For this review, take the finished solid that the model builds, in its own axes (mm). Face numbers are marked on the shaded views. A direction names the side the tool comes from. Coordinates: 2 decimals unless noted, no trailing zeros. Order: outer loops, then holes, each group sorted by start corner. A loop starts at its lowest first (then second) coordinate and runs counter-clockwise, first axis right, second up. Notation, with made-up numbers: M 29.25,11 L 82.25,11 A31 ccw 82.25,36 Z; hole C 26,48 d9. An arc over 180 degrees is marked long. Use CSV: the item, a comma, the result in double quotes.
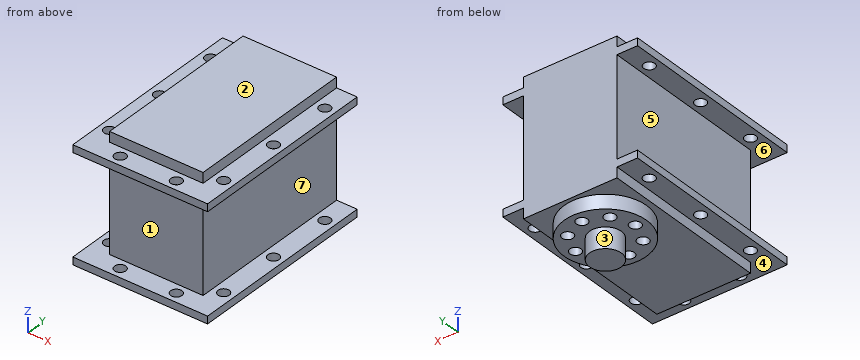
```python
from build123d import *

# Parameters (mm, degrees)
SKETCH1_W           = 25
SKETCH1_H           = 45.5
BOSS_EXTRUDE1_DEPTH = 36
BOSS_EXTRUDE2_START = -2.75
SKETCH2_W           = 36
SKETCH2_H           = 51
SKETCH2_R           = 1.5
BOSS_EXTRUDE2_DEPTH = 2
SKETCH3_R           = 11
BOSS_EXTRUDE3_DEPTH = 3.75
SKETCH4_R           = 1.5
CUT_EXTRUDE1_DEPTH  = 3.75
SKETCH5_R           = 4.25
BOSS_EXTRUDE4_DEPTH = 5.5
BOSS_EXTRUDE5_START = -4.75
SKETCH6_W           = 36
SKETCH6_H           = 51
SKETCH6_R           = 1.5
BOSS_EXTRUDE5_DEPTH = 2


with BuildPart() as part:
    # Sketch1 → Boss-Extrude1 (new body)
    with BuildSketch(Plane.XY):
        Rectangle(SKETCH1_W, SKETCH1_H)
    extrude(amount=BOSS_EXTRUDE1_DEPTH)

    # Sketch2 → Boss-Extrude2 (add)
    with BuildSketch(Plane(origin=(0, 0, 0), x_dir=(-1, 0, 0), z_dir=(0, 0, -1)).offset(BOSS_EXTRUDE2_START)):
        with Locations((0, -2.75)):
            Rectangle(SKETCH2_W, SKETCH2_H)
        with Locations((-15.25, 15.25)):
            Circle(SKETCH2_R, mode=Mode.SUBTRACT)
        with Locations((-15.25, -2.25)):
            Circle(SKETCH2_R, mode=Mode.SUBTRACT)
        with Locations((-15.25, -19.25)):
            Circle(SKETCH2_R, mode=Mode.SUBTRACT)
        with Locations((-7.5, -25.5)):
            Circle(SKETCH2_R, mode=Mode.SUBTRACT)
        with Locations((7.5, -25.5)):
            Circle(SKETCH2_R, mode=Mode.SUBTRACT)
        with Locations((15.25, -19.25)):
            Circle(SKETCH2_R, mode=Mode.SUBTRACT)
        with Locations((15.25, -2.25)):
            Circle(SKETCH2_R, mode=Mode.SUBTRACT)
        with Locations((15.25, 15.25)):
            Circle(SKETCH2_R, mode=Mode.SUBTRACT)
    extrude(amount=-BOSS_EXTRUDE2_DEPTH)

    # Sketch3 → Boss-Extrude3 (add)
    with BuildSketch(Plane(origin=(0, 0, 0), x_dir=(-1, 0, 0), z_dir=(0, 0, -1))):
        with Locations((0, 10.75)):
            Circle(SKETCH3_R)
    extrude(amount=BOSS_EXTRUDE3_DEPTH)

    # Sketch4 → Cut-Extrude1 (cut)
    with BuildSketch(Plane(origin=(0, 0, -3.75), x_dir=(-1, 0, 0), z_dir=(0, 0, -1))):
        with Locations((0, 18.75)):
            Circle(SKETCH4_R)
        with Locations((-5.656854249, 16.406854249)):
            Circle(SKETCH4_R)
        with Locations((-8, 10.75)):
            Circle(SKETCH4_R)
        with Locations((-5.656854249, 5.093145751)):
            Circle(SKETCH4_R)
        with Locations((0, 2.75)):
            Circle(SKETCH4_R)
        with Locations((5.656854249, 5.093145751)):
            Circle(SKETCH4_R)
        with Locations((8, 10.75)):
            Circle(SKETCH4_R)
        with Locations((5.656854249, 16.406854249)):
            Circle(SKETCH4_R)
    extrude(amount=-CUT_EXTRUDE1_DEPTH, mode=Mode.SUBTRACT)

    # Sketch5 → Boss-Extrude4 (add)
    with BuildSketch(Plane(origin=(0, 0, -3.75), x_dir=(-1, 0, 0), z_dir=(0, 0, -1))):
        with Locations((0, 10.75)):
            Circle(SKETCH5_R)
    extrude(amount=BOSS_EXTRUDE4_DEPTH)

    # Sketch6 → Boss-Extrude5 (add)
    with BuildSketch(Plane.XY.offset(36).offset(BOSS_EXTRUDE5_START)):
        with Locations((0, -2.75)):
            Rectangle(SKETCH6_W, SKETCH6_H)
        with Locations(Location((-15.25, 15.25, 0), (0, 0, 180))):
            Circle(SKETCH6_R, mode=Mode.SUBTRACT)
        with Locations(Location((-15.25, -2.25, 0), (0, 0, 180))):
            Circle(SKETCH6_R, mode=Mode.SUBTRACT)
        with Locations(Location((-15.25, -19.25, 0), (0, 0, 180))):
            Circle(SKETCH6_R, mode=Mode.SUBTRACT)
        with Locations(Location((-7.5, -25.5, 0), (0, 0, 180))):
            Circle(SKETCH6_R, mode=Mode.SUBTRACT)
        with Locations(Location((7.5, -25.5, 0), (0, 0, 180))):
            Circle(SKETCH6_R, mode=Mode.SUBTRACT)
        with Locations(Location((15.25, -19.25, 0), (0, 0, 180))):
            Circle(SKETCH6_R, mode=Mode.SUBTRACT)
        with Locations(Location((15.25, -2.25, 0), (0, 0, 180))):
            Circle(SKETCH6_R, mode=Mode.SUBTRACT)
        with Locations(Location((15.25, 15.25, 0), (0, 0, 180))):
            Circle(SKETCH6_R, mode=Mode.SUBTRACT)
    extrude(amount=BOSS_EXTRUDE5_DEPTH)


solid = part.part
```
Item 1: Draft analysis for pull direction Z (two halves, no side actions). For the marked faces 1, 2 and 3, state which applies: released by +Z, released by -Z, zero draft, split by the parting line, or undercut.
Solutions:
face 1,"undercut"
face 2,"released by +Z"
face 3,"zero draft"
Item 2: Clearance check with flat-ended pins moving along their axes: pin 1 Ø2.5 at (x, y) = (-15.25, 15.25) entering from -Z; pin 2 Ø3.5 at (x, y) = (-0.5, 2.5) entering from -Z; pin 3 Ø1.5 at (x, z) = (-13, 0.5) entering from -Y; pin 4 Ø1.5 at (x, y) = (6, 16) entering from -Z. State where each tip first meets the part, or that it passes through.
Solutions:
pin 1,"through"
pin 2,"z = -3.75"
pin 3,"y = -22.75"
pin 4,"z = 0"
Item 3: To check wall thickness, follow line 1 along Y through (x, z) = (15.25, 3.6); line 2 along X through (y, z) = (15.25, 32.65); line 3 along Z through (x, y) = (-15.5, -15). State the ranges of each line that lie inside material, in increasing order. Write a range as [from, to].
Solutions:
line 1,"[-28.25, -20.75], [-17.75, -3.75], [-0.75, 13.75], [16.75, 22.75]"
line 2,"[-18, -16.75], [-13.75, 13.75], [16.75, 18]"
line 3,"[2.75, 4.75], [31.25, 33.25]"
Item 4: For the marked faces 4, 5, 6 and 7, list the 3-axis set-ups (+Z, -Z, +X, -X, +Y, -Y) from which the entire face can be reached by the end or side of a thin tool; tool diameter is ignored.
Solutions:
face 4,"-Z, -Y"
face 5,"-X, +Y, -Y"
face 6,"-Y"
face 7,"+X, +Y, -Y"
Item 5: Add section B-B on y = -25.5. State the section outline as (x, z) points.
Solutions:
outline,"M -18,2.75 L -9,2.75 L -9,4.75 L -18,4.75 Z; M -18,31.25 L -9,31.25 L -9,33.25 L -18,33.25 Z; M -6,2.75 L 6,2.75 L 6,4.75 L -6,4.75 Z; M -6,31.25 L 6,31.25 L 6,33.25 L -6,33.25 Z; M 9,2.75 L 18,2.75 L 18,4.75 L 9,4.75 Z; M 9,31.25 L 18,31.25 L 18,33.25 L 9,33.25 Z"
Item 6: Add section A-A on x = -15.25. State how many separate pieces and enclosed holes the cut face has, and give its area (3 significant figures).
Solutions:
separate pieces,"8"
enclosed holes,"0"
area,"168 mm^2"
Item 7: Add section D-D on y = -11. State the section outline as (x, z) points.
Solutions:
outline,"M -18,2.75 L -12.5,2.75 L -12.5,0 L 12.5,0 L 12.5,2.75 L 18,2.75 L 18,4.75 L 12.5,4.75 L 12.5,31.25 L 18,31.25 L 18,33.25 L 12.5,33.25 L 12.5,36 L -12.5,36 L -12.5,33.25 L -18,33.25 L -18,31.25 L -12.5,31.25 L -12.5,4.75 L -18,4.75 Z"
